Read the model definition and answer for the solid it produces. Units are mm, in the model's axes. Round coordinates to 2 decimals unless told otherwise and drop trailing zeros. Loops run counter-clockwise (first coordinate to the right, second up) from the corner with the lowest first, then second, coordinate; pieces in that order, holes last. Notation, with made-up numbers: (-24.5, -17.75) -> (-2.5, -17.75) arc R36 ccw to (-2.5, 20.25) -> close; hole circle Ø5 at (63, 8.25). An arc over 180 degrees is marked (long way). Put each result on its own line as item: value.
from build123d import *

# Parameters (mm, degrees)
SKETCH1_W               = 40
SKETCH1_H               = 227
BOSS_EXTRUDE1_DEPTH     = 2
SKETCH2_W               = 10
SKETCH2_H               = 2
BOSS_EXTRUDE2_DEPTH     = 3
LPATTERN1_COUNT         = 2
LPATTERN1_PITCH         = 20
SKETCH3_W               = 10
SKETCH3_H               = 2
BOSS_EXTRUDE3_DEPTH     = 3
LPATTERN2_COUNT         = 2
LPATTERN2_PITCH         = 20
SKETCH4_W               = 2
SKETCH4_H               = 10
BOSS_EXTRUDE4_DEPTH     = 3
LPATTERN3_COUNT         = 12
LPATTERN3_PITCH         = 20
ESQUISSE1_W             = 3
ESQUISSE1_H             = 3
ENL_V_MAT_EXTRU_1_DEPTH = 3
ESQUISSE2_W             = 1
ESQUISSE2_H             = 227
ESQUISSE2_W_2           = 43
ESQUISSE2_H_2           = 1
BOSS_EXTRU_1_DEPTH      = 2


with BuildPart() as part:
    # Sketch1 → Boss-Extrude1 (new body)
    with BuildSketch(Plane.XY):
        with Locations((20, 113.5)):
            Rectangle(SKETCH1_W, SKETCH1_H)
    extrude(amount=BOSS_EXTRUDE1_DEPTH)

    # Sketch2 → Boss-Extrude2 (add)
    with BuildSketch(Plane.XZ):
        with Locations((25, 1)):
            Rectangle(SKETCH2_W, SKETCH2_H)
    boss_extrude2 = extrude(amount=BOSS_EXTRUDE2_DEPTH)

    # LPattern1: Boss-Extrude2 ×2
    with Locations(*[(-i * LPATTERN1_PITCH, 0, 0) for i in range(1, LPATTERN1_COUNT)]):
        add(boss_extrude2)

    # Sketch3 → Boss-Extrude3 (add)
    with BuildSketch(Plane(origin=(0, 227, 0), x_dir=(1, 0, 0), z_dir=(0, 1, 0))):
        with Locations((25, -1)):
            Rectangle(SKETCH3_W, SKETCH3_H)
    boss_extrude3 = extrude(amount=BOSS_EXTRUDE3_DEPTH)

    # LPattern2: Boss-Extrude3 ×2
    with Locations(*[(-i * LPATTERN2_PITCH, 0, 0) for i in range(1, LPATTERN2_COUNT)]):
        add(boss_extrude3)

    # Sketch4 → Boss-Extrude4 (add)
    with BuildSketch(Plane.ZY):
        with Locations((1, 5)):
            Rectangle(SKETCH4_W, SKETCH4_H)
    boss_extrude4 = extrude(amount=BOSS_EXTRUDE4_DEPTH)

    # LPattern3: Boss-Extrude4 ×12
    with Locations(*[(0, i * LPATTERN3_PITCH, 0) for i in range(1, LPATTERN3_COUNT)]):
        add(boss_extrude4)

    # Esquisse1 → Enlèv. mat.-Extru.1 (cut, through all)
    with BuildSketch(Plane.XY.offset(2)):
        with Locations((-1.5, 228.5)):
            Rectangle(ESQUISSE1_W, ESQUISSE1_H)
    extrude(amount=-ENL_V_MAT_EXTRU_1_DEPTH, mode=Mode.SUBTRACT)

    # Esquisse2 → Boss.-Extru.1 (add)
    with BuildSketch(Plane.XY.offset(2)):
        with Locations((-0.5, 113.5)):
            Rectangle(ESQUISSE2_W, ESQUISSE2_H)
        with Locations((18.5, -0.5)):
            Rectangle(ESQUISSE2_W_2, ESQUISSE2_H_2)
    extrude(amount=-BOSS_EXTRU_1_DEPTH)


solid = part.part
Item 1: The part is cut by section A-A (y = 72). Determine the outline of the cut face in (x, z), then the cut area to 3 significant figures.
Derived:
outline: (-1, 0) -> (40, 0) -> (40, 2) -> (-1, 2) -> close
area: 82.0 mm^2
Item 2: Flat-ended cylindrical pins translate along their axes: pin 1 Ø0.6 at (x, z) = (-2, 1) entering from +Y; pin 2 Ø0.6 at (y, z) = (229, 0.5) entering from -X. Find the tip coordinate at first contact, or state that the pin passes through.
Derived:
pin 1: stops at y = 227
pin 2: stops at x = 0
Item 3: Find the intervals of material crossed by line 1 along Y through (x, z) = (16, 1.1); line 2 along X through (y, z) = (96, 1.5), in increasing order.
Derived:
line 1: y = -1 to 227
line 2: x = -1 to 40
Item 4: The part is cut by section B-B (x = 17). Determine the outline of the cut face in (y, z), then the cut area to 3 significant figures.
Derived:
outline: (-1, 0) -> (227, 0) -> (227, 2) -> (-1, 2) -> close
area: 456 mm^2
